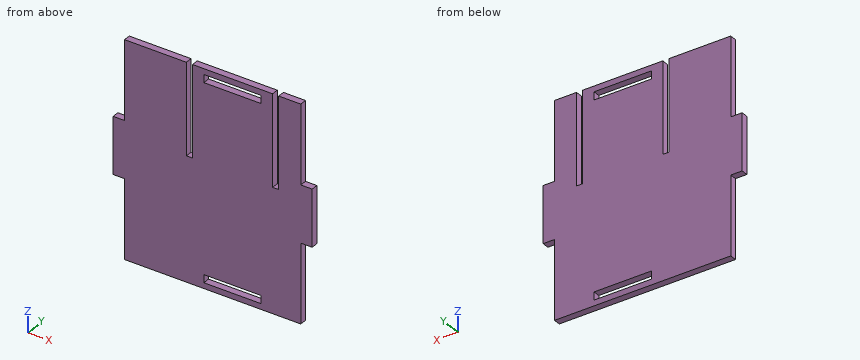
```python
from build123d import *

# Parameters (mm, degrees)
SKETCH1_W           = 50.4
SKETCH1_H           = 7
SKETCH1_W_2         = 10
SKETCH1_H_2         = 50
BOSS_EXTRUDE1_DEPTH = 6


with BuildPart() as part:
    # Sketch1 → Boss-Extrude1 (new body)
    with BuildSketch(Plane(origin=(0, 0, 0), x_dir=(1, 0, 0), z_dir=(0, 1, 0))):
        Polygon((-19.4, 0), (0, 0), (0, 69.5), (0, 119.5), (0, 189), (-155, 189), (-155, 119.5), (-155, 69.5), (-155, 0), (-100.6, 0), (-100.6, 80.4), (-95.2, 80.4), (-95.2, 0), (-75, 0), (-25, 0), (-24.8, 0), (-24.8, 80.4), (-19.4, 80.4), align=None)
        with Locations((-60, 8.5)):
            Rectangle(SKETCH1_W, SKETCH1_H, mode=Mode.SUBTRACT)
        with Locations((-60, 180.5)):
            Rectangle(SKETCH1_W, SKETCH1_H, mode=Mode.SUBTRACT)
        with Locations((-160, 94.5)):
            Rectangle(SKETCH1_W_2, SKETCH1_H_2)
        with Locations((5, 94.5)):
            Rectangle(SKETCH1_W_2, SKETCH1_H_2)
    extrude(amount=BOSS_EXTRUDE1_DEPTH)


solid = part.part
```
CAD build for the part. Positions are in the model's coordinates, mm. Round coordinates to 2 decimals unless told otherwise and drop trailing zeros. Write each loop counter-clockwise with the first axis right and the second up, starting at its lowest first coordinate (ties: lowest second). Pieces come first, ordered by that corner, then holes. Notation, with made-up numbers: (-26.5, -9) -> (10.5, -9) arc R13 ccw to (10.5, -1) -> close; hole circle Ø11 at (-8.5, -13.5). An arc over 180 degrees is marked (long way). Answer in a Markdown table with one row per item. Add a question column.
Item 1: Saw through at D-D, the plane z = -168. Write the cut outline in (x, y), then the cut area to 3 significant figures.
Item 2: Saw through at A-A, the plane z = -46. Write the cut outline in (x, y), then the cut area to 3 significant figures.
Item 3: Drill centre lines: line 1 (Z direction, x = -62, y = 0.3); line 2 (X direction, y = 0.4, z = -37.5); line 3 (X direction, y = 3.5, z = -8). Where is each one in solid material? Low to high. Write a range as from..to.
Item 4: Saw through at C-C, the plane x = -39.5. Write the cut outline in (y, z).
Item 5: Drop flat-ended pins along their axis: pin 1 Ø1.5 at (x, y) = (-22, 1) entering from +Z; pin 2 Ø1.8 at (x, y) = (-161, 4) entering from -Z; pin 3 Ø1.8 at (y, z) = (4, -32) entering from -X. Give the stop position or say it passes through.
Item 6: Saw through at B-B, the plane y = 3.3. Write the cut outline in (x, z), then the cut area to 3 significant figures.
Findings below:
| question | item | result |
|---|---|---|
| 1 | outline | (-155, 0) -> (0, 0) -> (0, 6) -> (-155, 6) -> close |
| 1 | area | 930 mm^2 |
| 2 | outline | (-155, 0) -> (-100.6, 0) -> (-100.6, 6) -> (-155, 6) -> close; (-95.2, 0) -> (-24.8, 0) -> (-24.8, 6) -> (-95.2, 6) -> close; (-19.4, 0) -> (0, 0) -> (0, 6) -> (-19.4, 6) -> close |
| 2 | area | 865 mm^2 |
| 3 | line 1 | z = -189..-184, -177..-12, -5..0 |
| 3 | line 2 | x = -155..-100.6, -95.2..-24.8, -19.4..0 |
| 3 | line 3 | x = -155..-100.6, -95.2..-85.2, -34.8..-24.8, -19.4..0 |
| 4 | outline | (0, -189) -> (6, -189) -> (6, -184) -> (0, -184) -> close; (0, -177) -> (6, -177) -> (6, -12) -> (0, -12) -> close; (0, -5) -> (6, -5) -> (6, 0) -> (0, 0) -> close |
| 5 | pin 1 | stops at z = -80.4 |
| 5 | pin 2 | stops at z = -119.5 |
| 5 | pin 3 | stops at x = -155 |
| 6 | outline | (-165, -119.5) -> (-155, -119.5) -> (-155, -189) -> (0, -189) -> (0, -119.5) -> (10, -119.5) -> (10, -69.5) -> (0, -69.5) -> (0, 0) -> (-19.4, 0) -> (-19.4, -80.4) -> (-24.8, -80.4) -> (-24.8, 0) -> (-95.2, 0) -> (-95.2, -80.4) -> (-100.6, -80.4) -> (-100.6, 0) -> (-155, 0) -> (-155, -69.5) -> (-165, -69.5) -> close; hole (-85.2, -184) -> (-34.8, -184) -> (-34.8, -177) -> (-85.2, -177) -> close; hole (-85.2, -12) -> (-34.8, -12) -> (-34.8, -5) -> (-85.2, -5) -> close |
| 6 | area | 28,700 mm^2 |
